```python
from build123d import *

# Parameters (mm, degrees)
BOX003_W                  = 15
BOX003_H                  = 3.4
BOX003_DEPTH              = 17
ARRAY_Y_COUNT             = 2
ARRAY_Y_PITCH             = 6
CYLINDER002_R             = 2.2
CYLINDER002_DEPTH         = 6
CYLINDER001_R             = 1.9
CYLINDER001_DEPTH         = 15
FUSION001_PLACEMENT_ANGLE = 90
CYLINDER_R                = 7.5
CYLINDER_DEPTH            = 19.6
BOX002_W                  = 15
BOX002_H                  = 19.6
BOX002_DEPTH              = 12.5
CYLINDER006_R             = 1.9
CYLINDER006_DEPTH         = 15
BOX007_W                  = 9
BOX007_H                  = 15
BOX007_DEPTH              = 15
BOX006_W                  = 15
BOX006_H                  = 15
BOX006_DEPTH              = 20


with BuildPart() as side_3_extract_cube_array:
    # Box003 → Box003 (new body)
    with BuildSketch(Plane(origin=(-7.5, -7.7, 3), x_dir=(1, 0, 0), z_dir=(0, 0, 1))):
        with Locations((7.5, 1.7)):
            Rectangle(BOX003_W, BOX003_H)
    extrude(amount=BOX003_DEPTH)

    # Array Y: side 3 extract cube array ×2


with BuildPart() as side_3_extract_cube_array_1:
    add(side_3_extract_cube_array.part)
    with Locations(*[(0, i * ARRAY_Y_PITCH, 0) for i in range(1, ARRAY_Y_COUNT)]):
        add(side_3_extract_cube_array.part)


with BuildPart() as side_3_extract_cube_array_2:
    # Array placement: moved
    add(side_3_extract_cube_array_1.part.moved(Location((0, 3, 0))))


with BuildPart() as insert_hole:
    # Cylinder002 → Cylinder002 (new body)
    with BuildSketch(Plane.XY):
        Circle(CYLINDER002_R)
    extrude(amount=CYLINDER002_DEPTH)


with BuildPart() as side_3_extract_fusion:
    # Cylinder001 → Cylinder001 (new body)
    with BuildSketch(Plane.XY.offset(6)):
        Circle(CYLINDER001_R)
    extrude(amount=CYLINDER001_DEPTH)

    # Fusion001: union insert hole
    add(insert_hole.part)


with BuildPart() as side_3_extract_fusion_1:
    # Fusion001 placement: moved
    add(side_3_extract_fusion.part.moved(Location((0, 11.1, 12.5))).rotate(Axis((0, 11.1, 12.5), (1, 0, 0)), FUSION001_PLACEMENT_ANGLE))

    # Fusion002: union side 3 extract cube array
    add(side_3_extract_cube_array_2.part)


with BuildPart() as outer_cylinder:
    # Cylinder → Cylinder (new body)
    with BuildSketch(Plane(origin=(0, 11.1, 12.5), x_dir=(1, 0, 0), z_dir=(0, -1, 0))):
        Circle(CYLINDER_R)
    extrude(amount=CYLINDER_DEPTH)


with BuildPart() as side_3_cut_clone001:
    # Box002 → Box002 (new body)
    with BuildSketch(Plane(origin=(-7.5, -8.5, 0), x_dir=(1, 0, 0), z_dir=(0, 0, 1))):
        with Locations((7.5, 9.8)):
            Rectangle(BOX002_W, BOX002_H)
    extrude(amount=BOX002_DEPTH)

    # Fusion: union outer cylinder
    add(outer_cylinder.part)

    # Cut: cut side 3 extract fusion
    add(side_3_extract_fusion_1.part, mode=Mode.SUBTRACT)


with BuildPart() as side_3_cut_clone001_1:
    # Body002 placement: moved
    add(side_3_cut_clone001.part.moved(Location((0, 0, 35))))


with BuildPart() as bolt_hole001:
    # Cylinder006 → Cylinder006 (new body)
    with BuildSketch(Plane(origin=(-7.5, 0, 7.5), x_dir=(0, 0, -1), z_dir=(1, 0, 0))):
        Circle(CYLINDER006_R)
    extrude(amount=CYLINDER006_DEPTH)


with BuildPart() as one_cube_with_bolt_hole:
    # Box007 → Box007 (new body)
    with BuildSketch(Plane(origin=(-1.5, -7.5, 0), x_dir=(1, 0, 0), z_dir=(0, 0, 1))):
        with Locations((4.5, 7.5)):
            Rectangle(BOX007_W, BOX007_H)
    extrude(amount=BOX007_DEPTH)

    # Cut002: cut bolt hole001
    add(bolt_hole001.part, mode=Mode.SUBTRACT)


with BuildPart() as side_3_one_fusion:
    # Box006 → Box006 (new body)
    with BuildSketch(Plane(origin=(-7.5, -7.5, 15), x_dir=(1, 0, 0), z_dir=(0, 0, 1))):
        with Locations((7.5, 7.5)):
            Rectangle(BOX006_W, BOX006_H)
    extrude(amount=BOX006_DEPTH)

    # Fusion005: union side 3 cut clone001, one cube with bolt hole
    add(side_3_cut_clone001_1.part)
    add(one_cube_with_bolt_hole.part)


solid = side_3_one_fusion.part
```
CAD build for the part. Positions are in the model's coordinates, mm. A direction names the side the tool comes from. Round coordinates to 2 decimals unless told otherwise and drop trailing zeros. Order: outer loops, then holes, each group sorted by start corner. A loop starts at its lowest first (then second) coordinate and runs counter-clockwise, first axis right, second up. Notation, with made-up numbers: (82.25, 33.25) - (87.25, 33.25) arc R13 cw to (87.25, 37.25) - close; hole circle Ø11 at (83.25, 77.5). An arc over 180 degrees is marked (long way). Answer as CSV lines item,"result". Start each with the question number.
1. Pin check, flat tips, straight feed: pin 1 (4.5 mm diameter, centred on y = 0, z = 7.5, fed in from +X); pin 2 (5 mm diameter, centred on x = 2.5, z = 22, fed in from +Y); pin 3 (2.5 mm diameter, centred on x = 0, y = 3, fed in from +Z); pin 4 (5 mm diameter, centred on x = -5.5, y = 0.5, fed in from -Z). Stop position of each tip, or through.
2. Drill centre lines: L1, parallel to Y at x = 2, z = 44; L2, parallel to X at y = -0.1, z = 47.5; L3, parallel to Y at x = 0.5, z = 45.5. Where is each one in solid material? Low to high. Write a range as [from, to].
3. Tool access for faces 1 (the face through (0, -1.3, 44)), 2 (the face through (0, 9, 35)), 3 (the face through (0, -8, 35)), 4 (the face through (0, -8.5, 45)): list every direction of +Z, -Z, +X, -X, +Y, -Y with a clear straight run to the whole face (end or side of a thin tool).
4. Saw through at C-C, the plane z = 7.5. Write the cut outline in (x, y).
5. Saw through at B-B, the plane y = 0. Write the cut outline in (x, z), and give its area (3 significant figures).
6. Pull direction Y, two halves, no side cores. Call faces 5 (the face through (-7.5, 1, 31)), 6 (the face through (0, -3, 38)), 7 (the face through (2, 7.5, 21)), 8 (the face through (2, -7.5, 21)): +Y half, -Y half, draft (parallel to the pull), parting line (faces both ways), or undercut.
7. Saw through at A-A, the plane x = 0. Count the separate pieces of the cut face and the enclosed holes in it, and give its area (3 significant figures).
8. Saw through at D-D, the plane y = 6. Write the cut outline in (x, z).
Model answer:
1,pin 1,"stops at x = 7.5"
1,pin 2,"stops at y = 7.5"
1,pin 3,"stops at z = 38"
1,pin 4,"stops at z = 15"
2,L1,"y = [-8.5, -4.7], [-1.3, 1.3], [4.7, 11.1]"
2,L2,"x = [-7.5, -1.9], [1.9, 7.5]"
2,L3,"y = [-8.5, -4.7], [-1.3, 1.3], [4.7, 5.1]"
3,face 1,"+Z, +X, -X"
3,face 2,"-Z, +X, -X, +Y"
3,face 3,"-Z, +X, -X, -Y"
3,face 4,"+Z, -Z, +X, -X, -Y"
4,outline,"(-1.5, -7.5) - (7.5, -7.5) - (7.5, -1.9) - (-1.5, -1.9) - close; (-1.5, 1.9) - (7.5, 1.9) - (7.5, 7.5) - (-1.5, 7.5) - close"
5,outline,"(-7.5, 15) - (-1.5, 15) - (-1.5, 9.4) - (7.5, 9.4) - (7.5, 47.5) arc R7.5 ccw to (-7.5, 47.5) - close; (-1.5, 0) - (7.5, 0) - (7.5, 5.6) - (-1.5, 5.6) - close; hole circle Ø3.8 at (0, 47.5)"
5,area,"665 mm²"
6,face 5,"draft"
6,face 6,"undercut"
6,face 7,"+Y half"
6,face 8,"-Y half"
7,separate pieces,"4"
7,enclosed holes,"1"
7,area,"738 mm²"
8,outline,"(-7.5, 15) - (-1.5, 15) - (-1.5, 0) - (7.5, 0) - (7.5, 47.5) arc R7.5 ccw to (-7.5, 47.5) - close; hole circle Ø4.4 at (0, 47.5)"
